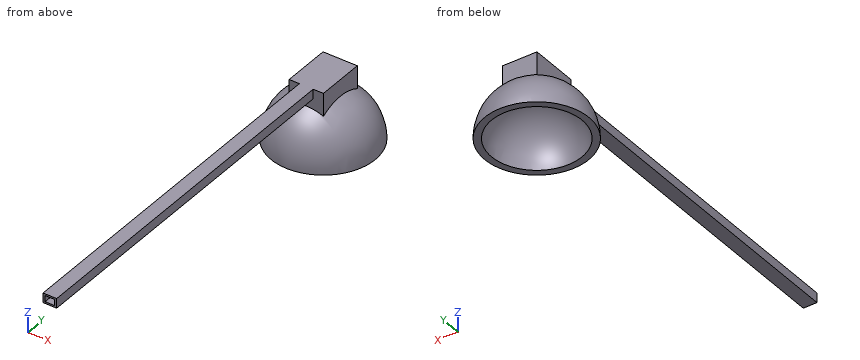
from build123d import *

# Parameters (mm, degrees)
REVOLVE1_ANGLE                  = 180
BOSS_EXTRUDE2_REACH             = 67.818
BOSS_EXTRUDE2_END_RADIUS        = 38
SKETCH2_W                       = 25
SKETCH2_H                       = 35
BOSS_EXTRUDE2_DIRECTION_2_DEPTH = 10
SKETCH5_W                       = 10
SKETCH5_H                       = 300
BOSS_EXTRUDE3_DEPTH             = 7
SKETCH6_W                       = 7
SKETCH6_H                       = 4.5
CUT_EXTRUDE1_DEPTH              = 265


with BuildPart() as part:
    # Sketch1 → Revolve1 (revolve)
    with BuildSketch(Plane.XY):
        with BuildLine():
            Line((0, 38), (0, 33))
            ThreePointArc((0, 33), (33, 0), (0, -33))
            Line((0, -33), (0, -38))
            ThreePointArc((0, -38), (38, 0), (0, 38))
        make_face()
    revolve(axis=Axis((0, -33, 0), (0, -1, 0)), revolution_arc=REVOLVE1_ANGLE)

    # Boss-Extrude2: up to this sphere (the profile starts outside it)
    boss_extrude2_end = Location((0, 0, 0)) * Sphere(BOSS_EXTRUDE2_END_RADIUS, mode=Mode.PRIVATE)
    # Sketch2 → Boss-Extrude2 (add, up to the surface)
    with BuildSketch(Plane(origin=(0, 0, 38), x_dir=(-1, 0, 0), z_dir=(0, 0, -1)), mode=Mode.PRIVATE) as boss_extrude2_sk1:
        Rectangle(SKETCH2_W, SKETCH2_H)
    boss_extrude2_tool1 = extrude(boss_extrude2_sk1.sketch, amount=BOSS_EXTRUDE2_REACH, mode=Mode.PRIVATE) - boss_extrude2_end
    add(boss_extrude2_tool1.solids().sort_by_distance((0, 0, 38))[0])

    # Sketch2 → Boss-Extrude2 direction 2 (add)
    with BuildSketch(Plane(origin=(0, 0, 38), x_dir=(-1, 0, 0), z_dir=(0, 0, -1))):
        Rectangle(SKETCH2_W, SKETCH2_H)
    extrude(amount=-BOSS_EXTRUDE2_DIRECTION_2_DEPTH)

    # Sketch5 → Boss-Extrude3 (add)
    with BuildSketch(Plane.XY.offset(48)):
        with Locations((0, -132.5)):
            Rectangle(SKETCH5_W, SKETCH5_H)
    extrude(amount=-BOSS_EXTRUDE3_DEPTH)

    # Sketch6 → Cut-Extrude1 (cut)
    with BuildSketch(Plane(origin=(0, -282.5, 0), x_dir=(-1, 0, 0), z_dir=(0, -1, 0))):
        with Locations((0, -44.5)):
            Rectangle(SKETCH6_W, SKETCH6_H)
    extrude(amount=-CUT_EXTRUDE1_DEPTH, mode=Mode.SUBTRACT)


solid = part.part
Read the model definition and answer for the solid it produces. Units are mm, in the model's axes. Coordinates: 2 decimals unless noted, no trailing zeros. Loops run counter-clockwise (first coordinate to the right, second up) from the corner with the lowest first, then second, coordinate; pieces in that order, holes last.
Q1. The part is cut by section C-C on z = 17. Write down the section's boundary in (x, y), and give its area (3 significant figures).
Q2. Consider probe 1 along Z at (x, y) = (2, -152.5); probe 2 along X at (y, z) = (-28, 43); probe 3 along X at (y, z) = (7, 21.5). Determine where each line is inside the solid, lowest interval first.
Q3. The part is cut by section B-B on y = -216.5. Write down the section's boundary in (x, z).
Q4. The part is cut by section D-D on x = -25. Write down the section's boundary in (y, z).
Q5. The part is cut by section A-A on y = -26. Write down the section's boundary in (x, z).
Q6. Each of these flat-tipped pins is pushed along its axis until it touches: pin 1 Ø5 at (x, z) = (3.5, 41) entering from +Y; pin 2 Ø12 at (x, z) = (-20, 26) entering from +Y; pin 3 Ø8.5 at (y, z) = (0.5, 41.5) entering from +X. Where does it stop, or does it pass through?
Results below:
1. outline: circle Ø67.97 at (0, 0); hole circle Ø56.57 at (0, 0)
1. area: 1,120 mm2
2. probe 1: z = 41 to 42.25, 46.75 to 48
2. probe 2: x = -5 to -3.5, 3.5 to 5
2. probe 3: x = -30.54 to -24.04, 24.04 to 30.54
3. outline: (-5, 41) - (5, 41) - (5, 48) - (-5, 48) - close; hole (-3.5, 42.25) - (3.5, 42.25) - (3.5, 46.75) - (-3.5, 46.75) - close
4. outline: (-28.62, 0) - (-21.54, 0) arc R21.54 cw to (21.54, 0) - (28.62, 0) arc R28.62 ccw to start
5. outline: (-27.71, 0) - (-20.32, 0) arc R20.32 cw to (20.32, 0) - (27.71, 0) arc R27.71 ccw to start; (-5, 41) - (5, 41) - (5, 48) - (-5, 48) - close; hole (-3.5, 42.25) - (3.5, 42.25) - (3.5, 46.75) - (-3.5, 46.75) - close
6. pin 1: stops at y = 17.5
6. pin 2: stops at y = 26.94
6. pin 3: stops at x = 12.5
